Input: part model. Units: mm. Frame: model coordinates. Face numbers are marked on the shaded views. Give positions to 0.01 mm unless a question says otherwise; leave off trailing zeros. Loops run counter-clockwise (first coordinate to the right, second up) from the corner with the lowest first, then second, coordinate; pieces in that order, holes last. Notation, with made-up numbers: M -12.75,73 L 37.25,73 A16 cw 37.25,77 Z; hole C 39.5,27 d11. An arc over 180 degrees is marked long. One line per item, written item: value. Start each with the question number.
(1) Pin query (flat end, axial travel): P1, Ø5, axis at x = -3.5, y = 2, coming from the -Z side. Return the tip coordinate at first contact, or that it passes through.
(2) Section A-A on z = 1.5. Output: boundary loops of the cut face in (x, y), plus the area to 3 significant figures.
(3) Ray query, line 1 along X through (y, z) = (-5, 0.6); line 2 along X through (y, z) = (4.75, 2.75); line 3 along Y through (x, z) = (3.5, 1.85). Return the intervals inside material, ascending. Write a range as from..to.
(4) Pull-direction query (Y, two-part tool) for the marked faces 1, 2 and 3; classes: released by +Y, released by -Y, zero draft, split by the parting line, or undercut.
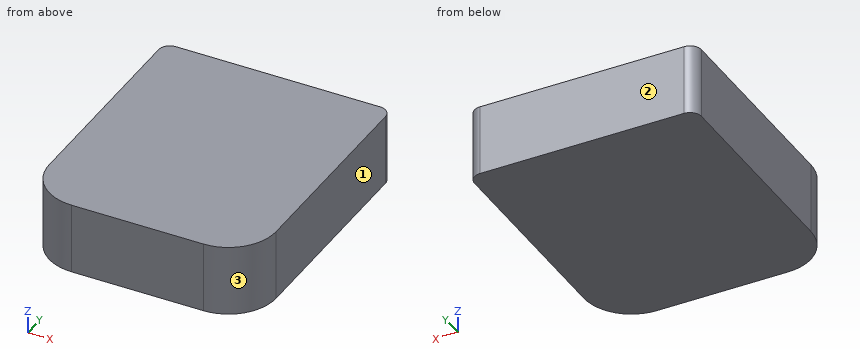
```python
from build123d import *

# Parameters (mm, degrees)
SKETCH1_W           = 10
SKETCH1_H           = 11.7
BOSS_EXTRUDE1_DEPTH = 3.125
FILLET1_R           = 2.1
FILLET2_R           = 0.5


with BuildPart() as part:
    # Sketch1 → Boss-Extrude1 (new body)
    with BuildSketch(Plane.XY):
        with Locations((0, -0.95)):
            Rectangle(SKETCH1_W, SKETCH1_H)
    extrude(amount=BOSS_EXTRUDE1_DEPTH)

    # Fillet1
    fillet1_edges = [part.edges().sort_by_distance(p)[0] for p in [
        (5, -6.8, 1.5625),
        (-5, -6.8, 1.5625),
    ]]
    fillet(fillet1_edges, radius=FILLET1_R)

    # Fillet2
    fillet2_edges = [part.edges().sort_by_distance(p)[0] for p in [
        (-5, 4.9, 1.5625),
        (5, 4.9, 1.5625),
    ]]
    fillet(fillet2_edges, radius=FILLET2_R)


solid = part.part
```
Output values:
1. P1: stops at z = 0
2. outline: M -5,-4.7 A2.1 ccw -2.9,-6.8 L 2.9,-6.8 A2.1 ccw 5,-4.7 L 5,4.4 A0.5 ccw 4.5,4.9 L -4.5,4.9 A0.5 ccw -5,4.4 Z
2. area: 115 mm²
3. line 1: x = -4.98..4.98
3. line 2: x = -4.86..4.86
3. line 3: y = -6.71..4.9
4. face 1: zero draft
4. face 2: released by +Y
4. face 3: released by -Y
